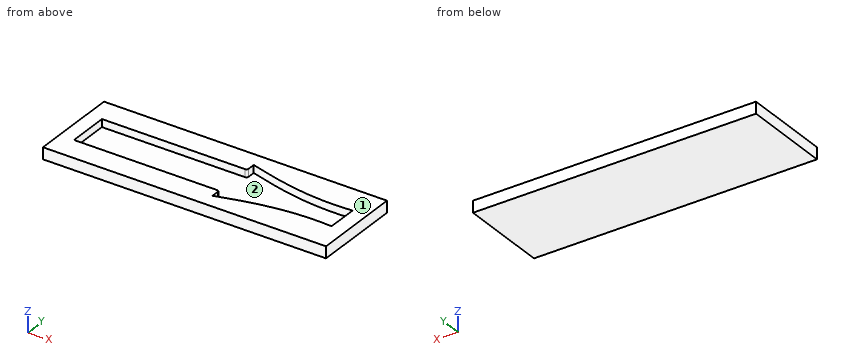
from build123d import *

# Parameters (mm, degrees)
SKETCH3_W           = 146.45
SKETCH3_H           = 46.142690012
BOSS_EXTRUDE1_DEPTH = 10
SKETCH5_W           = 146.45
SKETCH5_H           = 46.142690012
BOSS_EXTRUDE2_DEPTH = 6
BOSS_EXTRUDE3_DEPTH = 4


with BuildPart() as part:
    # Sketch3 → Boss-Extrude1 (new body)
    with BuildSketch(Plane.XY):
        with Locations((221.625, 0)):
            Rectangle(SKETCH3_W, SKETCH3_H)
        with BuildLine():
            Line((231.014073024, 15.571345006), (155.9, 15.571345006))
            Line((155.9, 15.571345006), (155.9, -15.571345006))
            Line((155.9, -15.571345006), (231.014073024, -15.571345006))
            add(Edge.make_bspline(
                [(231.014073024, -15.571345006), (235.603926114, -14.253380454), (240.202907461, -12.969220406), (247.161881801, -11.267037426), (249.489374332, -10.737991357), (254.165641768, -9.787213526), (256.514768348, -9.366822526), (263.601279745, -8.301427441), (268.338086531, -7.848826201), (275.456073059, -7.568289481), (277.831222276, -7.541362556), (282.586677642, -7.625574787), (284.967063297, -7.738842578), (287.35, -7.920409313)],
                knots=[0, 0, 0, 0, 0.25, 0.25, 0.375, 0.375, 0.5, 0.5, 0.75, 0.75, 0.875, 0.875, 1, 1, 1, 1], degree=3))
            Line((287.35, -7.920409313), (287.35, 7.920409313))
            add(Edge.make_bspline(
                [(287.35, 7.920409313), (284.969156465, 7.739002066), (282.587135429, 7.625484493), (277.820616166, 7.541273347), (275.436154733, 7.568458416), (268.279260355, 7.852389695), (263.532649453, 8.309357778), (256.45099394, 9.377629241), (254.104302816, 9.79880166), (249.438001237, 10.749341419), (247.117365, 11.277508342), (240.182218106, 12.975127096), (235.594114602, 14.256197804), (231.014073024, 15.571345006)],
                knots=[0, 0, 0, 0, 0.125, 0.125, 0.25, 0.25, 0.5, 0.5, 0.625, 0.625, 0.75, 0.75, 1, 1, 1, 1], degree=3))
        make_face(mode=Mode.SUBTRACT)
    extrude(amount=BOSS_EXTRUDE1_DEPTH)

    # Sketch5 → Boss-Extrude2 (add)
    with BuildSketch(Plane.XY):
        with Locations((221.625, 0)):
            Rectangle(SKETCH5_W, SKETCH5_H)
    extrude(amount=BOSS_EXTRUDE2_DEPTH)

    # Sketch6 → Boss-Extrude3 (add)
    with BuildSketch(Plane.XY.offset(6)):
        with BuildLine():
            Line((231.014073024, 15.571345006), (155.9, 15.571345006))
            Line((155.9, 15.571345006), (155.9, 10.571345006))
            Line((155.9, 10.571345006), (230.014073024, 10.571345006))
            ThreePointArc((230.014073024, 10.571345006), (230.721179805, 10.864238225), (231.014073024, 11.571345006))
            Line((231.014073024, 11.571345006), (231.014073024, 15.571345006))
        make_face()
        with BuildLine():
            Line((231.014073024, -15.571345006), (155.9, -15.571345006))
            Line((155.9, -15.571345006), (155.9, -10.571345006))
            Line((155.9, -10.571345006), (230.014073024, -10.571345006))
            ThreePointArc((230.014073024, -10.571345006), (230.721179805, -10.864238225), (231.014073024, -11.571345006))
            Line((231.014073024, -11.571345006), (231.014073024, -15.571345006))
        make_face()
    extrude(amount=BOSS_EXTRUDE3_DEPTH)

    # SurfaceCut2
    split(bisect_by=Plane.XY.offset(4), keep=Keep.TOP)


solid = part.part
The model under review builds one solid part; all positions refer to its coordinate system, in mm. Face numbers are marked on the shaded views. Give positions to 0.01 mm unless a question says otherwise; leave off trailing zeros. Order: outer loops, then holes, each group sorted by start corner. A loop starts at its lowest first (then second) coordinate and runs counter-clockwise, first axis right, second up. Notation, with made-up numbers: (78, 83.5) -> (117, 83.5) arc R24 cw to (117, 99.5) -> close; hole circle Ø2 at (22, -1.75). An arc over 180 degrees is marked (long way). Write item = value, one per line. Start each with the question number.
(1) Take a section at A-A (x = 218.5). Write out the cut boundary in (y, z).
(2) Take a section at B-B (y = 4). Write out the cut boundary in (x, z), plus the area to 3 significant figures.
(3) For L1, parallel to Y at x = 167.5, z = 9.5; L2, parallel to X at y = 1.5, z = 6.75; L3, parallel to Z at x = 216.5, y = -9.5, list the stretches that pass through material, from the lowest coordinate up. Write a range as from..to.
(4) For pin 1 Ø2 at (x, y) = (181, 0) entering from +Z, flat-tipped, find the tip position at first contact; note if it passes through.
(5) Draft analysis for pull direction Y (two halves, no side actions). For the marked faces 1 and 2, state which applies: +Y half, -Y half, draft (parallel to the pull), parting line (faces both ways), or undercut.
Returned:
q1.outline = (-23.07, 4) -> (23.07, 4) -> (23.07, 10) -> (10.57, 10) -> (10.57, 6) -> (-10.57, 6) -> (-10.57, 10) -> (-23.07, 10) -> close
q2.outline = (148.4, 4) -> (294.85, 4) -> (294.85, 10) -> (287.35, 10) -> (287.35, 6) -> (155.9, 6) -> (155.9, 10) -> (148.4, 10) -> close
q2.area = 353 mm²
q3.L1 = -23.07..-10.57, 10.57..23.07
q3.L2 = 148.4..155.9, 287.35..294.85
q3.L3 = 4..6
q4.pin_1 = 6
q5.face_1 = draft
q5.face_2 = undercut
